```python
from build123d import *

# Parameters (mm, degrees)
F0_R          = 17
F0_R_2        = 16
F0_R_3        = 14.45
F1_DEPTH      = 2.5
F2_DEPTH      = 1.5
F2_DEPTH_BACK = 1.5
F3_SIZE2      = 1.19999
F3_SIZE       = 1.54999
F4_SIZE       = 0.1
F6_SIZE       = 0.1


# Not quite as in the source:
# - a fillet or chamfer is up to 0.001 mm smaller than in the source, because OpenCascade refuses the exact size


with BuildPart() as f1:
    # F0 (on Top) → F1 (new body, symmetric)
    with BuildSketch(Plane.XY):
        Circle(F0_R)
        Circle(F0_R_2, mode=Mode.SUBTRACT)
        Circle(F0_R_2)
        Circle(F0_R_3, mode=Mode.SUBTRACT)
    extrude(amount=F1_DEPTH, both=True)

    # F0 (on Top) → F2 (cut, two sides)
    with BuildSketch(Plane.XY) as f2_sk:
        Circle(F0_R_2)
        Circle(F0_R_3, mode=Mode.SUBTRACT)
    extrude(amount=F2_DEPTH, mode=Mode.SUBTRACT)
    extrude(f2_sk.sketch, amount=-F2_DEPTH_BACK, mode=Mode.SUBTRACT)

    # F3 (size 1.55 and 1.2 in the source; OpenCascade refuses exactly that, so slightly less here)
    f3_edges = [f1.edges().sort_by_distance(p)[0] for p in [
        (-16, 0, -1.5),
        (-16, 0, 1.5),
    ]]
    chamfer(f3_edges, length=F3_SIZE, length2=F3_SIZE2)

    # F4
    f4_edges = [f1.edges().sort_by_distance(p)[0] for p in [
        (-17, 0, 2.5),
        (-17, 0, -2.5),
    ]]
    chamfer(f4_edges, length=F4_SIZE)

    # F6
    f6_edges = [f1.edges().sort_by_distance(p)[0] for p in [
        (-14.45, 0, 2.5),
        (-14.45, 0, -2.5),
    ]]
    chamfer(f6_edges, length=F6_SIZE)


solid = f1.part
```
Design review of the part built by this model. Coordinates are the model's own, in mm. A direction names the side the tool comes from. Coordinates: 2 decimals unless noted, no trailing zeros. Answer as a JSON object with one key per item and string values. Group by question number.
1) Wall thickness on L1, parallel to Y at x = 0, z = -0.2; L2, parallel to Y at x = 0, z = 1.75; L3, parallel to X at y = 1.5, z = 2.2: over which ranges is each line inside the solid? List them lowest first.
2) Tool access review of faces 4 (the conical face through (13.9, 4.4, -1.4)), 5 (the cylindrical face through (7.768, 12.184, -1.956)): name each direction out of +Z, -Z, +X, -X, +Y, -Y from which nothing blocks a thin tool from reaching the whole face with its end or side.
3) Mouldability with a two-part tool opening along X and no side actions: class faces 1 (the cylindrical face through (9.139, 14.334, 0.034)), 2 (the conical face through (13.9, 4.4, 1.4)), 3 (the flat face through (7, 13, 2.5)) as pulls with the +X half, pulls with the -X half, needs draft (parallel to the pull), parting line crosses it, or undercut.
4) For pin 1 (1.5 mm diameter, centred on y = -13, z = 0, fed in from +X); pin 2 (2 mm diameter, centred on y = 7, z = 0.5, fed in from +X), all flat-tipped, find the tip position at first contact; note any pin that passes through.
Computed values:
{
 "1": {"L1": "y = -17 to -16, 16 to 17", "L2": "y = -17 to -14.45, 14.45 to 17", "L3": "x = -16.93 to -14.37, 14.37 to 16.93"},
 "2": {"face 4": "none", "face 5": "+Z, -Z"},
 "3": {"face 1": "parting line crosses it", "face 2": "undercut", "face 3": "needs draft"},
 "4": {"pin 1": "stops at x = 11.79", "pin 2": "stops at x = 15.91"}
}
